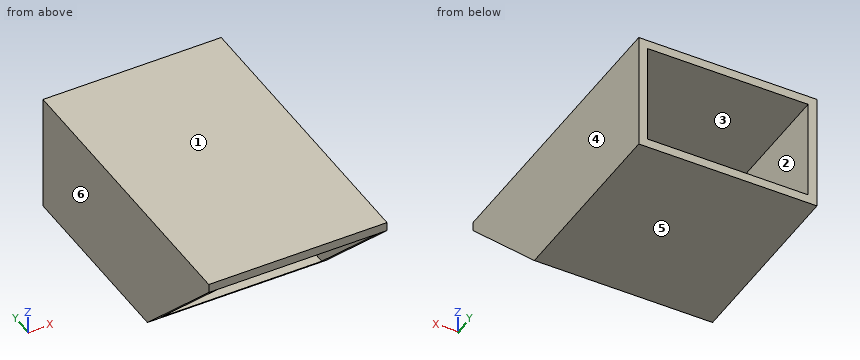
from build123d import *

# Parameters (mm, degrees)
F0_W     = 60
F0_H     = 100
F1_DEPTH = 40
F2_W     = 54
F2_H     = 34
F3_DEPTH = 141
F5_DEPTH = 60


with BuildPart() as f1:
    # F0 (on Top) → F1 (new body)
    with BuildSketch(Plane.XY):
        Rectangle(F0_W, F0_H)
    extrude(amount=F1_DEPTH)

    # F2 (on face) → F3 (cut)
    with BuildSketch(Plane.XZ.offset(50)):
        with Locations((0, 20)):
            Rectangle(F2_W, F2_H)
    extrude(amount=-F3_DEPTH, mode=Mode.SUBTRACT)

    # F4 (on face) → F5 (cut)
    with BuildSketch(Plane(origin=(-30, 0, 0), x_dir=(0, -1, 0), z_dir=(-1, 0, 0))):
        Polygon((50, 37), (13, 0), (50, 0), align=None)
    extrude(amount=-F5_DEPTH, mode=Mode.SUBTRACT)


solid = f1.part
CAD build for the part. Positions are in the model's coordinates, mm. Face numbers are marked on the shaded views. A direction names the side the tool comes from. Coordinates: 2 decimals unless noted, no trailing zeros. Write each loop counter-clockwise with the first axis right and the second up, starting at its lowest first coordinate (ties: lowest second). Pieces come first, ordered by that corner, then holes. Notation, with made-up numbers: (42, 48) - (96, 48) arc R35 ccw to (96, 81) - close; hole circle Ø7 at (80, 45.25). An arc over 180 degrees is marked (long way). Use a Markdown table: item, result. Add a question column.
Item 1: Band-saw the part on B-B, the plane z = 33.5. Give the cut face in (x, y), and give its area (3 significant figures).
Item 2: Band-saw the part on A-A, the plane x = -10. Give the cut face in (y, z), and give its area (4 significant figures).
Item 3: Drill centre lines: L1, parallel to X at y = 2, z = 4; L2, parallel to Z at x = -20, y = 40; L3, parallel to Z at x = 7.5, y = -43.5. Where is each one in solid material? Low to high. Write a range as from..to.
Item 4: 3-axis set-ups, long thin cutter, end or side, ignore diameter. For the marked faces 1 and 2: which of +Z, -Z, +X, -X, +Y, -Y reach the whole face in a straight line?
Item 5: Mould opens along X. For the marked faces 3, 4, 5 and 6 say: pulls with the +X half, pulls with the -X half, needs draft (parallel to the pull), parting line crosses it, or undercut.
Item 6: Band-saw the part on C-C, the plane y = 4. Give the cut face in (x, z), and give its area (3 significant figures).
Numbers:
| question | item | result |
|---|---|---|
| 1 | outline | (-30, -46.5) - (-27, -46.5) - (-27, 50) - (-30, 50) - close; (27, -46.5) - (30, -46.5) - (30, 50) - (27, 50) - close |
| 1 | area | 579 mm2 |
| 2 | outline | (-50, 37) - (50, 37) - (50, 40) - (-50, 40) - close; (-16, 3) - (-13, 0) - (50, 0) - (50, 3) - close |
| 2 | area | 493.5 mm2 |
| 3 | L1 | -30..-27, 27..30 |
| 3 | L2 | 0..3, 37..40 |
| 3 | L3 | 37..40 |
| 4 | face 1 | +Z, +X, -X, +Y, -Y |
| 4 | face 2 | +Y, -Y |
| 5 | face 3 | undercut |
| 5 | face 4 | pulls with the +X half |
| 5 | face 5 | needs draft |
| 5 | face 6 | pulls with the -X half |
| 6 | outline | (-30, 0) - (30, 0) - (30, 40) - (-30, 40) - close; hole (-27, 3) - (27, 3) - (27, 37) - (-27, 37) - close |
| 6 | area | 564 mm2 |
